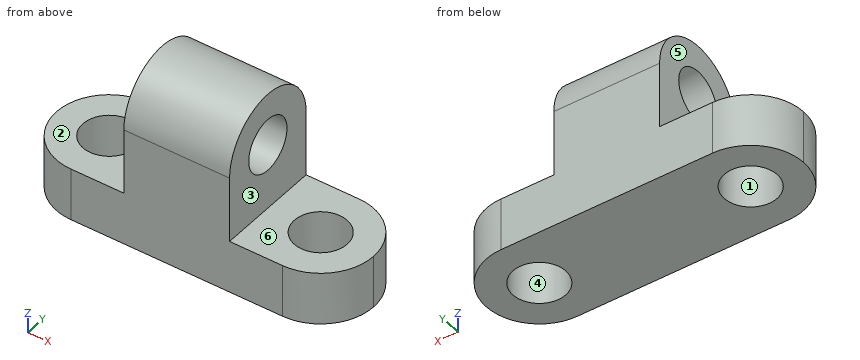
```python
from build123d import *

# Parameters (mm, degrees)
F1_DEPTH  = 25.4
F3_DEPTH  = 25.4
F4_R      = 6.35
F5_DEPTH  = 25.4
F7_DEPTH  = 25.4
F9_DEPTH  = 25.4
F10_R     = 6.35
F11_DEPTH = 25.4
F12_R     = 6.35
F13_DEPTH = 25.4


with BuildPart() as f1:
    # F0 (on Front) → F1 (new body)
    with BuildSketch(Plane.XZ):
        Polygon((-33.770596805, 12.7), (-33.770596805, 0), (42.429403195, 0), (42.429403195, 12.7), (17.029403195, 12.7), (17.029403195, 44.45), (-8.370596805, 44.45), (-8.370596805, 12.7), align=None)
    extrude(amount=F1_DEPTH)

    # F2 (on face) → F3 (cut)
    with BuildSketch(Plane.YZ.offset(17.029403195)):
        with BuildLine():
            ThreePointArc((-25.4, 28.575), (-12.7, 41.275), (0, 28.575))
            Line((0, 28.575), (0, 44.45))
            Line((0, 44.45), (-25.4, 44.45))
            Line((-25.4, 44.45), (-25.4, 28.575))
        make_face()
    extrude(amount=-F3_DEPTH, mode=Mode.SUBTRACT)

    # F4 (on face) → F5 (cut)
    with BuildSketch(Plane.YZ.offset(17.029403195)):
        with Locations((-12.7, 28.575)):
            Circle(F4_R)
    extrude(amount=-F5_DEPTH, mode=Mode.SUBTRACT)

    # F6 (on face) → F7 (cut)
    with BuildSketch(Plane.XY.offset(12.7)):
        with BuildLine():
            ThreePointArc((29.729403195, 0), (38.7096593161, -3.7197438789), (42.429403195, -12.7))
            Line((42.429403195, -12.7), (42.429403195, 0))
            Line((42.429403195, 0), (29.729403195, 0))
        make_face()
        with BuildLine():
            Line((42.429403195, -25.4), (42.429403195, -12.7))
            ThreePointArc((42.429403195, -12.7), (38.7096593161, -21.6802561211), (29.729403195, -25.4))
            Line((29.729403195, -25.4), (42.429403195, -25.4))
        make_face()
    extrude(amount=-F7_DEPTH, mode=Mode.SUBTRACT)

    # F8 (on face) → F9 (cut)
    with BuildSketch(Plane.XY.offset(12.7)):
        with BuildLine():
            ThreePointArc((-33.770596805, -12.7), (-30.0508529261, -3.7197438789), (-21.070596805, 0))
            Line((-21.070596805, 0), (-33.770596805, 0))
            Line((-33.770596805, 0), (-33.770596805, -12.7))
        make_face()
        with BuildLine():
            Line((-33.770596805, -25.4), (-21.070596805, -25.4))
            ThreePointArc((-21.070596805, -25.4), (-30.0508529261, -21.6802561211), (-33.770596805, -12.7))
            Line((-33.770596805, -12.7), (-33.770596805, -25.4))
        make_face()
    extrude(amount=-F9_DEPTH, mode=Mode.SUBTRACT)

    # F10 (on face) → F11 (cut)
    with BuildSketch(Plane.XY.offset(12.7)):
        with Locations((-21.070596805, -12.7)):
            Circle(F10_R)
    extrude(amount=-F11_DEPTH, mode=Mode.SUBTRACT)

    # F12 (on face) → F13 (cut)
    with BuildSketch(Plane.XY.offset(12.7)):
        with Locations((29.729403195, -12.7)):
            Circle(F12_R)
    extrude(amount=-F13_DEPTH, mode=Mode.SUBTRACT)


solid = f1.part
```
Source: CAD feature listing. Evaluate the final solid. Frame: model axes, mm. Face numbers are marked on the shaded views. A direction names the side the tool comes from. Give positions to 0.01 mm unless a question says otherwise; leave off trailing zeros. Loops run counter-clockwise (first coordinate to the right, second up) from the corner with the lowest first, then second, coordinate; pieces in that order, holes last. Notation, with made-up numbers: (74.25, -8.5) -> (123.25, -8.5) arc R14 cw to (123.25, 9.5) -> close; hole circle Ø11 at (-40, -23). An arc over 180 degrees is marked (long way). Use a Markdown table: item, result. Add a question column.
(1) Access query for the marked faces 4, 5 and 6. Directions: +Z, -Z, +X, -X, +Y, -Y. A direction counts if a zero-diameter tool reaches every point of the face in a straight line with its end or side. Return the directions, or none.
(2) Ray query, line 1 (X direction, y = -14.75, z = 3); line 2 (Z direction, x = 20.5, y = -8.75); line 3 (X direction, y = -12.25, z = 19). Return the intervals inside material, ascending.
(3) Pull-direction query (X, two-part tool) for the marked faces 1, 2 and 3; classes: +X half, -X half, draft (parallel to the pull), parting line (faces both ways), or undercut.
(4) Section query B-B (y = -7.25). Output: boundary loops of the cut face in (x, z).
(5) First-contact query: pin 1 Ø7.5 at (y, z) = (-15.5, 22.5) entering from -X; pin 2 Ø5 at (y, z) = (-11, 28) entering from +X; pin 3 Ø6 at (x, y) = (34.5, -19.5) entering from +Z; pin 4 Ø8 at (y, z) = (-19.5, 18.5) entering from +X. Flat tips, straight axial feed; report the tip coordinate or a pass-through.
(6) Section query C-C (x = 2.5). Output: boundary loops of the cut face in (y, z) (3 decimals), then the cut area to 3 significant figures.
(7) Section query D-D (z = 24). Output: boundary loops of the cut face in (x, y), then the cut area to 3 significant figures.
(8) Section query A-A (z = 4.5). Output: boundary loops of the cut face in (x, y).
Checked values:
| question | item | result |
|---|---|---|
| 1 | face 4 | +Z, -Z |
| 1 | face 5 | +Z, -X, +Y, -Y |
| 1 | face 6 | +Z, +X, +Y, -Y |
| 2 | line 1 | -33.6 to -27.08, -15.06 to 23.72, 35.74 to 42.26 |
| 2 | line 2 | 0 to 12.7 |
| 2 | line 3 | -8.37 to 17.03 |
| 3 | face 1 | undercut |
| 3 | face 2 | draft |
| 3 | face 3 | +X half |
| 4 | outline | (-32.54, 0) -> (-24.33, 0) -> (-24.33, 12.7) -> (-32.54, 12.7) -> close; (-17.81, 0) -> (26.47, 0) -> (26.47, 12.7) -> (17.03, 12.7) -> (17.03, 25.32) -> (-8.37, 25.32) -> (-8.37, 12.7) -> (-17.81, 12.7) -> close; (-8.37, 31.83) -> (17.03, 31.83) -> (17.03, 40.05) -> (-8.37, 40.05) -> close; (32.99, 0) -> (41.2, 0) -> (41.2, 12.7) -> (32.99, 12.7) -> close |
| 5 | pin 1 | x = -8.37 |
| 5 | pin 2 | through |
| 5 | pin 3 | z = 12.7 |
| 5 | pin 4 | x = 17.03 |
| 6 | outline | (-25.4, 0) -> (0, 0) -> (0, 28.575) arc R12.7 ccw to (-25.4, 28.575) -> close; hole circle Ø12.7 at (-12.7, 28.575) |
| 6 | area | 852 mm^2 |
| 7 | outline | (-8.37, -25.4) -> (17.03, -25.4) -> (17.03, -17.1) -> (-8.37, -17.1) -> close; (-8.37, -8.3) -> (17.03, -8.3) -> (17.03, 0) -> (-8.37, 0) -> close |
| 7 | area | 421 mm^2 |
| 8 | outline | (-21.07, -25.4) -> (29.73, -25.4) arc R12.7 ccw to (29.73, 0) -> (-21.07, 0) arc R12.7 ccw to start; hole circle Ø12.7 at (-21.07, -12.7); hole circle Ø12.7 at (29.73, -12.7) |
